Build history of the part. All positions in model axes, mm. Round coordinates to 2 decimals unless told otherwise and drop trailing zeros. Order: outer loops, then holes, each group sorted by start corner. A loop starts at its lowest first (then second) coordinate and runs counter-clockwise, first axis right, second up. Notation, with made-up numbers: (30.25, 29) -> (76.25, 29) arc R35 cw to (76.25, 64) -> close; hole circle Ø6 at (64.5, -19). An arc over 180 degrees is marked (long way). Answer as a JSON object with one key per item and string values.
Autodesk Inventor part; units mm, degrees
ref_plane "YZ Plane" through (0, 0, 0) normal (1, 0, 0) x (0, 1, 0)
ref_plane "XZ Plane" through (0, 0, 0) normal (0, 1, 0) x (-1, 0, 0)
ref_plane "XY Plane" through (0, 0, 0) normal (0, 0, 1) x (1, 0, 0)
sketch "Sketch1" plane through (0, 0, 0) normal (0, 0, 1) x (1, 0, 0)
  line L0 (-55, 43.25) -> (55, 43.25)
  line L1 (55, 43.25) -> (55, -43.25)
  line L2 (55, -43.25) -> (-55, -43.25)
  line L3 (-55, -43.25) -> (-55, 43.25)
  circle A0 centre (-39, 39.75) radius 1.55
  circle A1 centre (-51.5, -39.75) radius 1.55
  circle A2 centre (43.5, 35.75) radius 1.55
  circle A3 centre (51.5, -39.75) radius 1.55
  point P0 (0, 0)
  point P1 (-55, 0)
  point P2 (0, 43.25)
  dimension "d0" = 110
  dimension "d1" = 86.5
  dimension "d2" = 16
  dimension "d3" = 83
  dimension "d4" = 3.5
  dimension "d5" = 3.5
  dimension "d6" = 98.5
  dimension "d7" = 79
  dimension "d8" = 106.5
  dimension "d9" = 3.5
  dimension "d10" = 3.1
  dimension "d11" = 3.1
  dimension "d12" = 3.1
  dimension "d13" = 3.1
extrude "Extrusion1" add sketch "Sketch1" along normal blind 25
properties part number "udoomountingholes"
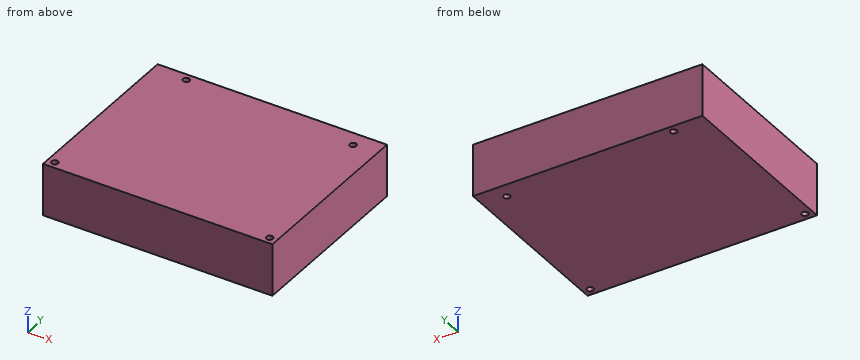
1) Cut at C-C, the plane y = 35.75. Give the cut face in (x, z).
Checked values:
{"outline": "(-55, 0) -> (41.95, 0) -> (41.95, 25) -> (-55, 25) -> close; (45.05, 0) -> (55, 0) -> (55, 25) -> (45.05, 25) -> close"}
2) Probe L1, parallel to Y at x = 43.5, z = 10.75; L2, parallel to Y at x = 51.5, z = 6.5. List the from-to ranges inside material, lowest first. Write a range as from..to.
Checked values:
{"L1": "y = -43.25..34.2, 37.3..43.25", "L2": "y = -43.25..-41.3, -38.2..43.25"}
3) Cut at B-B, the plane y = -39.75. Give the cut face in (x, z), plus the area to 4 significant figures.
Checked values:
{"outline": "(-55, 0) -> (-53.05, 0) -> (-53.05, 25) -> (-55, 25) -> close; (-49.95, 0) -> (49.95, 0) -> (49.95, 25) -> (-49.95, 25) -> close; (53.05, 0) -> (55, 0) -> (55, 25) -> (53.05, 25) -> close", "area": "2,595 mm²"}
4) Cut at A-A, the plane x = -39. Give the cut face in (y, z), plus the area to 4 significant figures.
Checked values:
{"outline": "(-43.25, 0) -> (38.2, 0) -> (38.2, 25) -> (-43.25, 25) -> close; (41.3, 0) -> (43.25, 0) -> (43.25, 25) -> (41.3, 25) -> close", "area": "2,085 mm²"}
